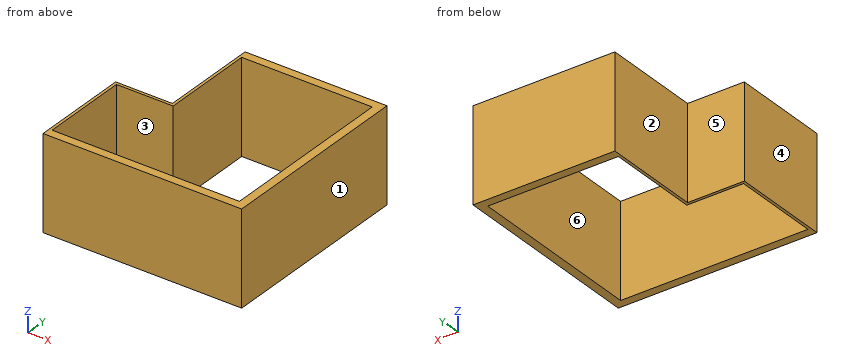
from build123d import *

# Parameters (mm, degrees)
F1_DEPTH      = 30
F1_DEPTH_BACK = 3


with BuildPart() as f1:
    # F0 (on Top) → F1 (new body, two sides)
    with BuildSketch(Plane.XY) as f1_sk:
        Polygon((0, 35), (0, 0), (3, 0), (70, 0), (70, 70), (20, 70), (20, 35), align=None)
        Polygon((67, 3), (3, 3), (1, 3), (1, 34), (21, 34), (21, 67), (67, 67), align=None, mode=Mode.SUBTRACT)
    extrude(amount=F1_DEPTH)
    extrude(f1_sk.sketch, amount=-F1_DEPTH_BACK)


solid = f1.part
Geometry: final body of the model. Coordinates: model frame, mm. Face numbers are marked on the shaded views. A direction names the side the tool comes from. Coordinates: 2 decimals unless noted, no trailing zeros. Loops run counter-clockwise (first coordinate to the right, second up) from the corner with the lowest first, then second, coordinate; pieces in that order, holes last. Notation, with made-up numbers: (-25.75, 65.25) - (-3.75, 65.25) arc R24 ccw to (-3.75, 102.25) - close; hole circle Ø7 at (-1.75, 53). An arc over 180 degrees is marked (long way). One line per question, with ' | ' between items. Start each with the question number.
(1) Draft query along X for the marked faces 1, 2 and 3. Return one class per face: +X half, -X half, draft (parallel to the pull), parting line (faces both ways), or undercut.
(2) Ray query, L1, parallel to Y at x = 39.5, z = 8.5; L2, parallel to X at y = 4.5, z = 1.5; L3, parallel to X at y = 54.5, z = 0. Return the intervals inside material, ascending. Write a range as from..to.
(3) First-contact query: pin 1 (8 mm diameter, centred on x = 14, y = 45, fed in from +Z); pin 2 (2 mm diameter, centred on x = 9.5, z = 10, fed in from +Y). Flat tips, straight axial feed; report the tip coordinate or a pass-through.
(4) Reachability of the marked faces 4, 5 and 6 from +Z, -Z, +X, -X, +Y, -Y: full face, straight path, thin tool, end or side. Return the list, or none.
(5) Cut plane C-C on z = 21. Output: boundary loops of the cut face in (x, y), and give its area (3 significant figures).
(6) Cut plane A-A on x = 25. Output: boundary loops of the cut face in (y, z), and give its area (3 significant figures).
(7) Cut plane B-B on y = 53.5. Output: boundary loops of the cut face in (x, z).
Here are the results:
1) face 1: +X half | face 2: -X half | face 3: undercut
2) L1: 0..3, 67..70 | L2: 0..1, 67..70 | L3: 20..21, 67..70
3) pin 1: through | pin 2: y = 35
4) face 4: +Z, -Z, -X, +Y, -Y | face 5: +Z, -Z, -X, +Y | face 6: +Z, -Z
5) outline: (0, 0) - (70, 0) - (70, 70) - (20, 70) - (20, 35) - (0, 35) - close; hole (1, 3) - (67, 3) - (67, 67) - (21, 67) - (21, 34) - (1, 34) - close | area: 636 mm²
6) outline: (0, -3) - (3, -3) - (3, 30) - (0, 30) - close; (67, -3) - (70, -3) - (70, 30) - (67, 30) - close | area: 198 mm²
7) outline: (20, -3) - (21, -3) - (21, 30) - (20, 30) - close; (67, -3) - (70, -3) - (70, 30) - (67, 30) - close
